```python
from build123d import *

# Parameters (mm, degrees)
F1_DEPTH = 63.5
F2_R     = 5.08
F3_R     = 5.881823
F4_DEPTH = 25.4


with BuildPart() as f1:
    # F0 (on Front) → F1 (new body, symmetric)
    with BuildSketch(Plane.XZ):
        Polygon((-16.709963, 12.094708), (-16.709963, -3.979688), (9.303563, -10.605776), (8.690037, 12.094708), align=None)
    extrude(amount=F1_DEPTH, both=True)

    # F2
    f2_edges = [f1.edges().sort_by_distance(p)[0] for p in [
        (-16.709963, 0, 12.094708),
    ]]
    fillet(f2_edges, radius=F2_R)

    # F3 (on face) → F4 (cut)
    with BuildSketch(Plane.XY.offset(12.094708)):
        with Locations((0, 30.291276)):
            Circle(F3_R)
    extrude(amount=-F4_DEPTH, mode=Mode.SUBTRACT)


solid = f1.part
```
Could you check a few things on this model? Use its own coordinates, in mm. Round coordinates to 2 decimals unless told otherwise and drop trailing zeros. Loops run counter-clockwise (first coordinate to the right, second up) from the corner with the lowest first, then second, coordinate; pieces in that order, holes last.
Q1. For P1, Ø4, axis at y = 50.5, z = -1, coming from the +X side; P2, Ø5, axis at x = -8.5, y = 51, coming from the -Z side; P3, Ø4, axis at x = 6, y = 36.5, coming from the -Z side, each with a flat end and sliding along its axis, tell me the tip position at first contact or that it passes through.
Q2. Thinking about a two-plate mould opening in Y: for faces 1 (the flat face through (-4, -63.5, 3)), 2 (the cylindrical face through (5.61, 32.06, 1.33)), 3 (the flat face through (-4, 63.5, 3)), 4 (the flat face through (-3.885, -0.889, -7.246)), which applies, pulls with the +Y half, pulls with the -Y half, needs draft (parallel to the pull), parting line crosses it, or undercut?
Q3. I want a section at D-D (z = -7.25). Write out the boundary of the cut face in (x, y).
Q4. I want a section at C-C (z = 5). Write out the boundary of the cut face in (x, y), and give its area (3 significant figures).
Q5. I want a section at A-A (x = -1.5). Write out the boundary of the cut face in (y, z).
Q6. Please list where these lines run through material, in increasing order: L1, parallel to Y at x = 0, z = -3.5; L2, parallel to Z at x = -9.25, y = 8.5; L3, parallel to X at y = 26, z = 0.
Q7. I want a section at B-B (y = 23). Write out the boundary of the cut face in (x, z).
Answer below:
1. P1: stops at x = 9.1
1. P2: stops at z = -6.71
1. P3: stops at z = -10.27
2. face 1: pulls with the -Y half
2. face 2: undercut
2. face 3: pulls with the +Y half
2. face 4: needs draft
3. outline: (-3.87, -63.5) - (9.21, -63.5) - (9.21, 63.5) - (-3.87, 63.5) - (-3.87, 34.72) arc R5.88 cw (long way) to (-3.87, 25.86) - close
4. outline: (-16.71, -63.5) - (8.88, -63.5) - (8.88, 63.5) - (-16.71, 63.5) - close; hole circle Ø11.76 at (0, 30.29)
4. area: 3,140 mm2
5. outline: (-63.5, -7.85) - (24.6, -7.85) - (24.6, 12.09) - (-63.5, 12.09) - close; (35.98, -7.85) - (63.5, -7.85) - (63.5, 12.09) - (35.98, 12.09) - close
6. L1: y = -63.5 to 24.41, 36.17 to 63.5
6. L2: z = -5.88 to 12.09
6. L3: x = -16.71 to -4.02, 4.02 to 9.02
7. outline: (-16.71, -3.98) - (9.3, -10.61) - (8.69, 12.09) - (-11.63, 12.09) arc R5.08 ccw to (-16.71, 7.01) - close
